Can you work these out from the model? Positions are in its coordinate system, mm. Face numbers are marked on the shaded views. Coordinates: 2 decimals unless noted, no trailing zeros. Order: outer loops, then holes, each group sorted by start corner. A loop starts at its lowest first (then second) coordinate and runs counter-clockwise, first axis right, second up. Notation, with made-up numbers: (68.5, 74) -> (115.5, 74) arc R23 ccw to (115.5, 111) -> close; hole circle Ø8 at (-24, 8). An arc over 180 degrees is marked (long way). Answer as CSV lines item,"result".
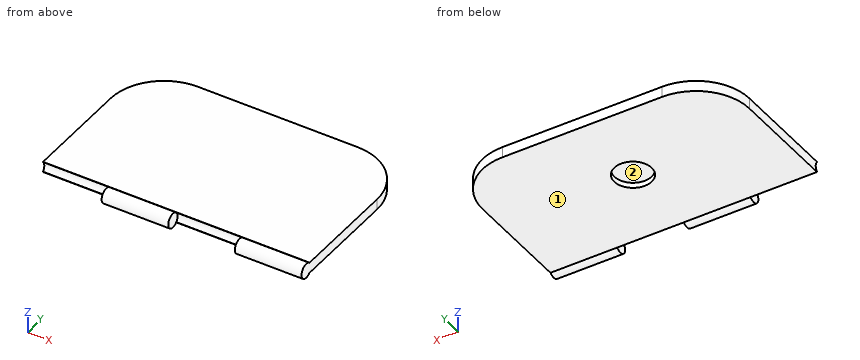
from build123d import *

# Parameters (mm, degrees)
BOSS_EXTRUDE1_DEPTH = 2
SKETCH3_R           = 1.375
CUT_EXTRUDE1_DEPTH  = 50
SKETCH3_2_R         = 1.375
BOSS_EXTRUDE2_DEPTH = 12.5
SKETCH5_R           = 1.375
BOSS_EXTRUDE3_DEPTH = 12.5
SKETCH7_R           = 3.5
CUT_EXTRUDE2_DEPTH  = 1


with BuildPart() as part:
    # Sketch1 → Boss-Extrude1 (new body)
    with BuildSketch(Plane.XY):
        with BuildLine():
            Line((-15, 15), (15, 15))
            ThreePointArc((15, 15), (22.071067812, 12.071067812), (25, 5))
            Line((25, 5), (25, -15))
            Line((25, -15), (-25, -15))
            Line((-25, -15), (-25, 5))
            ThreePointArc((-25, 5), (-22.071067812, 12.071067812), (-15, 15))
        make_face()
    extrude(amount=BOSS_EXTRUDE1_DEPTH)

    # Sketch3 → Cut-Extrude1 (cut)
    with BuildSketch(Plane(origin=(25, 0, 0), x_dir=(0, 0, -1), z_dir=(1, 0, 0))):
        with Locations((-1, -16)):
            Circle(SKETCH3_R)
    extrude(amount=-CUT_EXTRUDE1_DEPTH, mode=Mode.SUBTRACT)

    # Sketch3<2> → Boss-Extrude2 (add)
    with BuildSketch(Plane(origin=(25, 0, 0), x_dir=(0, 0, -1), z_dir=(1, 0, 0))):
        with Locations((-1, -16)):
            Circle(SKETCH3_2_R)
    extrude(amount=-BOSS_EXTRUDE2_DEPTH)

    # Sketch5 → Boss-Extrude3 (add)
    with BuildSketch(Plane.ZY):
        with Locations((1, -16)):
            Circle(SKETCH5_R)
    extrude(amount=BOSS_EXTRUDE3_DEPTH)

    # Sketch7 → Cut-Extrude2 (cut)
    with BuildSketch(Plane(origin=(0, 0, 0), x_dir=(-1, 0, 0), z_dir=(0, 0, -1))):
        Circle(SKETCH7_R)
    extrude(amount=-CUT_EXTRUDE2_DEPTH, mode=Mode.SUBTRACT)


solid = part.part
Q1. Imagine slicing it at A-A (y = -16). List the corners of the cut face in (x, z) for me (3 decimals).
Solution:
outline,"(-12.5, -0.375) -> (0, -0.375) -> (0, 2.375) -> (-12.5, 2.375) -> close; (12.5, -0.375) -> (25, -0.375) -> (25, 2.375) -> (12.5, 2.375) -> close"
Q2. Imagine slicing it at C-C (x = -4). List the corners of the cut face in (y, z) for me (3 decimals), and give its area (3 significant figures).
Solution:
outline,"(-15, 0) -> (15, 0) -> (15, 2) -> (-15, 2) -> (-15, 1.944) arc R1.375 ccw (long way) to (-15, 0.056) -> close"
area,"65.5 mm2"
Q3. For P1, Ø3, axis at x = 0.5, y = 9, coming from the +Z side; P2, Ø1.5, axis at x = 0.5, y = 4.5, coming from the -Z side; P3, Ø2, axis at x = 0, y = 1.5, coming from the -Z side; P4, Ø6, axis at x = 15.5, y = -13, coming from the -Z side (3 decimals), each with a flat end and sliding along its axis, tell me the tip position at first contact or that it passes through.
Solution:
P1,"z = 2"
P2,"z = 0"
P3,"z = 1"
P4,"z = -0.375"
Q4. We'd pull the mould along Y, two halves only. Please class the marked faces 1 and 2: pulls with the +Y half, pulls with the -Y half, needs draft (parallel to the pull), parting line crosses it, or undercut.
Solution:
face 1,"needs draft"
face 2,"undercut"
Q5. Imagine slicing it at D-D (x = 1). List the corners of the cut face in (y, z) for me (3 decimals).
Solution:
outline,"(-15, 0) -> (-3.354, 0) -> (-3.354, 1) -> (3.354, 1) -> (3.354, 0) -> (15, 0) -> (15, 2) -> (-15, 2) -> (-15, 1.944) arc R1.375 cw to (-15, 0.056) -> close"
Q6. If I drill on line 1 (Z direction, x = -21.5, y = 2); line 2 (Z direction, x = 2, y = 1); line 3 (X direction, y = 1, z = 0.95), over which ranges is the centre line in solid material (lowest first)?
Solution:
line 1,"0 to 2"
line 2,"1 to 2"
line 3,"-25 to -3.35, 3.35 to 25"
Q7. Imagine slicing it at B-B (y = 0). List the corners of the cut face in (x, z) for me, and give its area (3 significant figures).
Solution:
outline,"(-25, 0) -> (-3.5, 0) -> (-3.5, 1) -> (3.5, 1) -> (3.5, 0) -> (25, 0) -> (25, 2) -> (-25, 2) -> close"
area,"93.0 mm2"
